For this review, take the finished solid that the model builds, in its own axes (mm). Coordinates: 2 decimals unless noted, no trailing zeros. Loops run counter-clockwise (first coordinate to the right, second up) from the corner with the lowest first, then second, coordinate; pieces in that order, holes last. Notation, with made-up numbers: M -24,-28.75 L 3,-28.75 A8 cw 3,-14.75 Z; hole C 15.25,80 d3. An arc over 180 degrees is marked long. Write item = value, one per line.
from build123d import *

# Parameters (mm, degrees)
CYLINDER_R        = 2
CYLINDER_DEPTH    = 10
CYLINDER168_R     = 2
CYLINDER168_DEPTH = 10
CYLINDER169_R     = 2
CYLINDER169_DEPTH = 10
CYLINDER170_R     = 2
CYLINDER170_DEPTH = 10
CYLINDER171_R     = 2
CYLINDER171_DEPTH = 10
CYLINDER166_R     = 0.9
CYLINDER166_DEPTH = 1.3
CYLINDER165_R     = 0.9
CYLINDER165_DEPTH = 1.3
CYLINDER167_R     = 0.9
CYLINDER167_DEPTH = 1.3
CYLINDER164_R     = 0.9
CYLINDER164_DEPTH = 1.3
CYLINDER163_R     = 0.9
CYLINDER163_DEPTH = 1.3
BOX_W             = 24.5
BOX_H             = 1.3
BOX_DEPTH         = 36.5


with BuildPart() as cylinder:
    # Cylinder → Cylinder (new body)
    with BuildSketch(Plane(origin=(-3, 2, 14), x_dir=(1, 0, 0), z_dir=(0, -1, 0))):
        Circle(CYLINDER_R)
    extrude(amount=CYLINDER_DEPTH)


with BuildPart() as cylinder168:
    # Cylinder168 → Cylinder168 (new body)
    with BuildSketch(Plane(origin=(-14.5, 2, 14), x_dir=(1, 0, 0), z_dir=(0, -1, 0))):
        Circle(CYLINDER168_R)
    extrude(amount=CYLINDER168_DEPTH)


with BuildPart() as cylinder169:
    # Cylinder169 → Cylinder169 (new body)
    with BuildSketch(Plane(origin=(-21.5, 2, 14), x_dir=(1, 0, 0), z_dir=(0, -1, 0))):
        Circle(CYLINDER169_R)
    extrude(amount=CYLINDER169_DEPTH)


with BuildPart() as cylinder170:
    # Cylinder170 → Cylinder170 (new body)
    with BuildSketch(Plane(origin=(-3, 2, -16.5), x_dir=(1, 0, 0), z_dir=(0, -1, 0))):
        Circle(CYLINDER170_R)
    extrude(amount=CYLINDER170_DEPTH)


with BuildPart() as cylinder171:
    # Cylinder171 → Cylinder171 (new body)
    with BuildSketch(Plane(origin=(-21.5, 2, -16.5), x_dir=(1, 0, 0), z_dir=(0, -1, 0))):
        Circle(CYLINDER171_R)
    extrude(amount=CYLINDER171_DEPTH)


with BuildPart() as cylinder166:
    # Cylinder166 → Cylinder166 (new body)
    with BuildSketch(Plane(origin=(-14.62, 1.3, -17), x_dir=(1, 0, 0), z_dir=(0, -1, 0))):
        Circle(CYLINDER166_R)
    extrude(amount=CYLINDER166_DEPTH)


with BuildPart() as cylinder165:
    # Cylinder165 → Cylinder165 (new body)
    with BuildSketch(Plane(origin=(-12.08, 1.3, -17), x_dir=(1, 0, 0), z_dir=(0, -1, 0))):
        Circle(CYLINDER165_R)
    extrude(amount=CYLINDER165_DEPTH)


with BuildPart() as cylinder167:
    # Cylinder167 → Cylinder167 (new body)
    with BuildSketch(Plane(origin=(-17.16, 1.3, -17), x_dir=(1, 0, 0), z_dir=(0, -1, 0))):
        Circle(CYLINDER167_R)
    extrude(amount=CYLINDER167_DEPTH)


with BuildPart() as cylinder164:
    # Cylinder164 → Cylinder164 (new body)
    with BuildSketch(Plane(origin=(-9.54, 1.3, -17), x_dir=(1, 0, 0), z_dir=(0, -1, 0))):
        Circle(CYLINDER164_R)
    extrude(amount=CYLINDER164_DEPTH)


with BuildPart() as pcb_cutouts:
    # Cylinder163 → Cylinder163 (new body)
    with BuildSketch(Plane(origin=(-7, 1.3, -17), x_dir=(1, 0, 0), z_dir=(0, -1, 0))):
        Circle(CYLINDER163_R)
    extrude(amount=CYLINDER163_DEPTH)

    # Fusion: union Cylinder166, Cylinder165, Cylinder167, Cylinder164
    add(cylinder166.part)
    add(cylinder165.part)
    add(cylinder167.part)
    add(cylinder164.part)

    # Fusion001: union Cylinder, Cylinder168, Cylinder169, Cylinder170, Cylinder171
    add(cylinder.part)
    add(cylinder168.part)
    add(cylinder169.part)
    add(cylinder170.part)
    add(cylinder171.part)


with BuildPart() as pcb:
    # Box → Box (new body)
    with BuildSketch(Plane(origin=(-24.5, 0, -19.5), x_dir=(1, 0, 0), z_dir=(0, 0, 1))):
        with Locations((12.25, 0.65)):
            Rectangle(BOX_W, BOX_H)
    extrude(amount=BOX_DEPTH)

    # Cut: cut pcb cutouts
    add(pcb_cutouts.part, mode=Mode.SUBTRACT)


solid = pcb.part
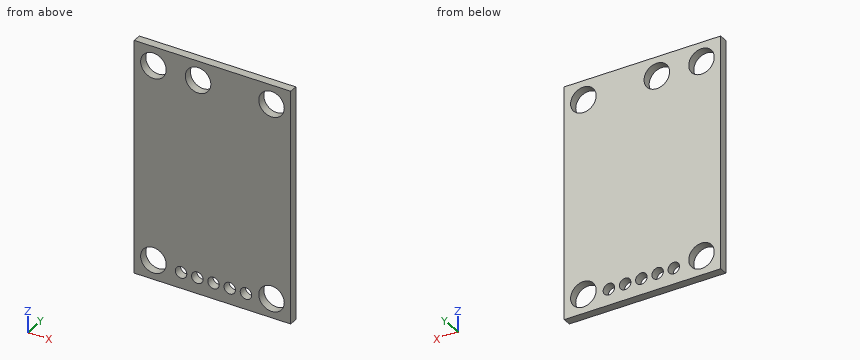
Q1. Add section C-C (x = -7). Write out the cut boundary in (y, z).
Solved:
outline = M 0,-19.5 L 1.3,-19.5 L 1.3,-17.9 L 0,-17.9 Z; M 0,-16.1 L 1.3,-16.1 L 1.3,17 L 0,17 Z
Q2. Add section B-B (y = 0.5). State how many separate pieces and enclosed holes the cut face has, and give its area (3 significant figures).
Solved:
separate_pieces = 1
enclosed_holes = 10
area = 819 mm²
Q3. Add section A-A (x = -3). Write out the cut boundary in (y, z).
Solved:
outline = M 0,-19.5 L 1.3,-19.5 L 1.3,-18.5 L 0,-18.5 Z; M 0,-14.5 L 1.3,-14.5 L 1.3,12 L 0,12 Z; M 0,16 L 1.3,16 L 1.3,17 L 0,17 Z
Q4. For line 1 along X through (y, z) = (1, 14); line 2 along Z through (x, y) = (-21.5, 0.35); line 3 along Z through (x, y) = (-14.5, 0.85), list the stretches that pass through material, from the lowest coordinate up.
Solved:
line_1 = -24.5 to -23.5, -19.5 to -16.5, -12.5 to -5, -1 to 0
line_2 = -19.5 to -18.5, -14.5 to 12, 16 to 17
line_3 = -19.5 to -17.89, -16.11 to 12, 16 to 17
